CAD build for the part. Positions are in the model's coordinates, mm. A direction names the side the tool comes from. Round coordinates to 2 decimals unless told otherwise and drop trailing zeros. Loops run counter-clockwise (first coordinate to the right, second up) from the corner with the lowest first, then second, coordinate; pieces in that order, holes last. Notation, with made-up numbers: (-16.5, 86.5) - (24.5, 86.5) arc R29 ccw to (24.5, 122.5) - close; hole circle Ø2 at (40.5, -12.75). An arc over 180 degrees is marked (long way). Use one line per item in the form item = value.
from build123d import *

# Parameters (mm, degrees)
SKETCH2_R           = 4.5
BOSS_EXTRUDE1_DEPTH = 20
SKETCH3_R           = 3
CUT_EXTRUDE1_DEPTH  = 10
SKETCH4_R           = 2.5
CUT_EXTRUDE2_DEPTH  = 10


with BuildPart() as part:
    # Sketch2 → Boss-Extrude1 (new body)
    with BuildSketch(Plane(origin=(0, 0, 0), x_dir=(1, 0, 0), z_dir=(0, 1, 0))):
        Circle(SKETCH2_R)
    extrude(amount=BOSS_EXTRUDE1_DEPTH)

    # Sketch3 → Cut-Extrude1 (cut)
    with BuildSketch(Plane(origin=(0, 20, 0), x_dir=(1, 0, 0), z_dir=(0, 1, 0))):
        Circle(SKETCH3_R)
    extrude(amount=-CUT_EXTRUDE1_DEPTH, mode=Mode.SUBTRACT)

    # Sketch4 → Cut-Extrude2 (cut)
    with BuildSketch(Plane.XZ):
        Circle(SKETCH4_R)
    extrude(amount=-CUT_EXTRUDE2_DEPTH, mode=Mode.SUBTRACT)


solid = part.part
1) Drill centre lines: probe 1 along Z at (x, y) = (0, 13.5); probe 2 along Z at (x, y) = (0, 4.75). Where is each one in solid material? Low to high.
Report:
probe_1 = -4.5 to -3, 3 to 4.5
probe_2 = -4.5 to -2.5, 2.5 to 4.5
2) Tool access for faces 1 (the flat face through (-2, 10, -2)), 2 (the flat face through (2, 0, 2)): list every direction of +Z, -Z, +X, -X, +Y, -Y with a clear straight run to the whole face (end or side of a thin tool).
Report:
face_1 = +Y
face_2 = +Z, -Z, +X, -X, -Y
3) Flat gauge pins, fed straight in: pin 1 (2 mm diameter, centred on x = 2, z = 0.5, fed in from +Y); pin 2 (1 mm diameter, centred on y = 10, z = 3, fed in from +X). Where does each tip first touch, or does it go through?
Report:
pin_1 = 20
pin_2 = 3.74
4) Slice it at C-C (y = 16). Write the cut outline in (x, z).
Report:
outline = circle Ø9 at (0, 0); hole circle Ø6 at (0, 0)
5) Slice it at D-D (x = 3.75). Write the cut outline in (y, z), plus the area to 3 significant figures.
Report:
outline = (0, -2.49) - (20, -2.49) - (20, 2.49) - (0, 2.49) - close
area = 99.5 mm^2
6) Slice it at A-A (x = 0). Write the cut outline in (y, z).
Report:
outline = (0, -4.5) - (20, -4.5) - (20, -3) - (10, -3) - (10, -2.5) - (0, -2.5) - close; (0, 2.5) - (10, 2.5) - (10, 3) - (20, 3) - (20, 4.5) - (0, 4.5) - close
7) Slice it at B-B (z = 0). Write the cut outline in (x, y).
Report:
outline = (-4.5, 0) - (-2.5, 0) - (-2.5, 10) - (-3, 10) - (-3, 20) - (-4.5, 20) - close; (2.5, 0) - (4.5, 0) - (4.5, 20) - (3, 20) - (3, 10) - (2.5, 10) - close
8) Two-plate mould, pull along X, no slides. Class faces 3 (the flat face through (1, 20, 3)), 4 (the cylindrical face through (-0.54, 4.93, -2.44)), 5 (the cylindrical face through (-0.59, 9.86, -4.46)): +X half, -X half, draft (parallel to the pull), parting line (faces both ways), or undercut.
Report:
face_3 = draft
face_4 = undercut
face_5 = parting line
